Geometry check sheet. Reference: drawing and pictorial views, mm from the part's lowest x, y, z. A direction names the side the tool comes from. Round coordinates to 2 decimals unless told otherwise and drop trailing zeros. Loops run counter-clockwise (first coordinate to the right, second up) from the corner with the lowest first, then second, coordinate; pieces in that order, holes last. Notation, with made-up numbers: (-9, 39.5) -> (10, 39.5) arc R17 ccw to (10, 71.5) -> close; hole circle Ø5 at (77.5, 32.5). An arc over 180 degrees is marked (long way). Write item = value, one per line.
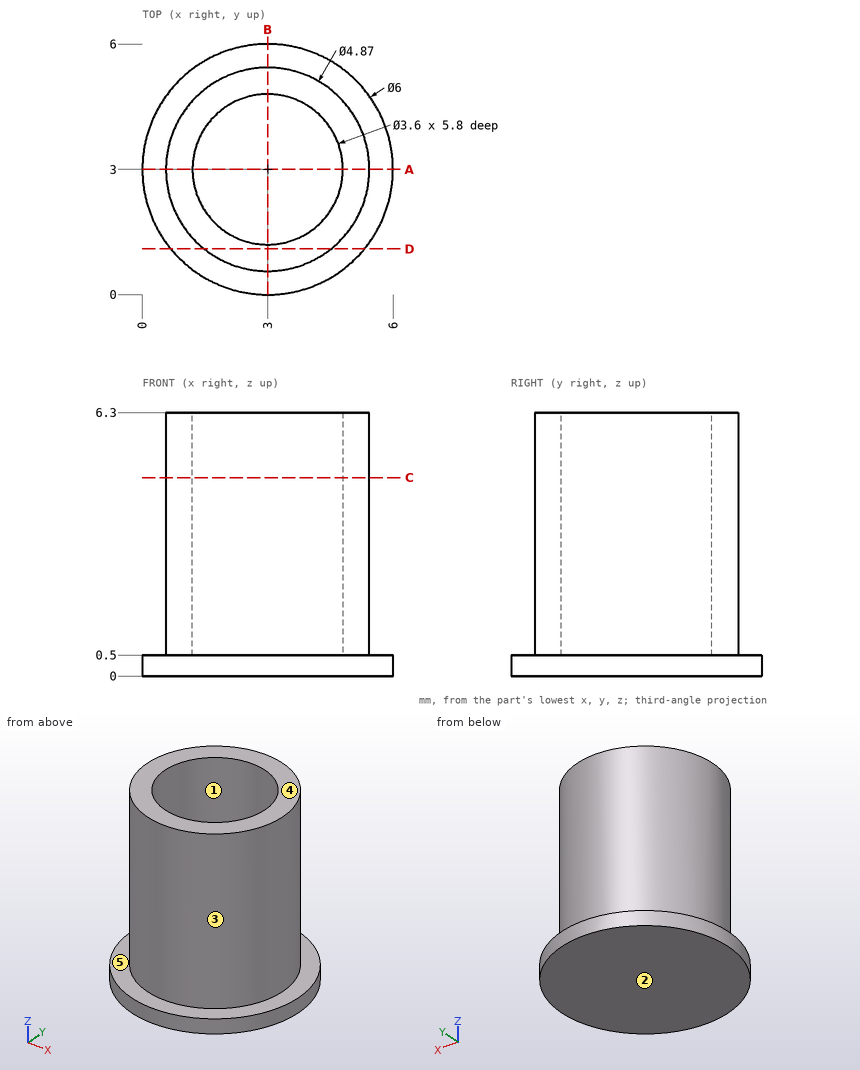
(1) Sectioned sample at D-D, the plane y = 1.1. Record the cut outline in (x, z).
Filled sheet:
outline = (0.68, 0) -> (5.32, 0) -> (5.32, 0.5) -> (4.52, 0.5) -> (4.52, 6.3) -> (1.48, 6.3) -> (1.48, 0.5) -> (0.68, 0.5) -> close
(2) Go/stop test with flat-tipped pins: pin 1 Ø1.5 at (x, y) = (3.5, 3) entering from +Z; pin 2 Ø3 at (y, z) = (5.5, 3.5) entering from -X; pin 3 Ø3 at (x, z) = (1, 5) entering from -Y. Record where each tip stops, or that it passes through.
Filled sheet:
pin_1 = 0.5
pin_2 = 0.78
pin_3 = 0.62
(3) Sectioned sample at C-C, the plane z = 4.75. Record the cut outline in (x, y) (3 decimals).
Filled sheet:
outline = circle Ø4.87 at (3, 3); hole circle Ø3.6 at (3, 3)
(4) Sectioned sample at A-A, the plane y = 3. Record the cut outline in (x, z) (3 decimals).
Filled sheet:
outline = (0, 0) -> (6, 0) -> (6, 0.5) -> (5.435, 0.5) -> (5.435, 6.3) -> (4.8, 6.3) -> (4.8, 0.5) -> (1.2, 0.5) -> (1.2, 6.3) -> (0.565, 6.3) -> (0.565, 0.5) -> (0, 0.5) -> close
(5) Draft check along X on the marked faces 1, 2 and 3. Enter one of: released by +X, released by -X, zero draft, split by the parting line, or undercut.
Filled sheet:
face_1 = undercut
face_2 = zero draft
face_3 = split by the parting line
(6) Material ranges on probe 1 along Y at (x, z) = (3, 1.7) (3 decimals); probe 2 along Z at (x, y) = (4.8, 1.05); probe 3 along X at (y, z) = (1.75, 1.75), recorded low to high. Write a range as from..to.
Filled sheet:
probe_1 = 0.565..1.2, 4.8..5.435
probe_2 = 0..0.5
probe_3 = 0.91..1.7, 4.3..5.09
(7) Set-up check for the marked faces 4 and 5: record each of +Z, -Z, +X, -X, +Y, -Y from which the full face is reachable in a straight line by a thin tool's end or side.
Filled sheet:
face_4 = +Z, +X, -X, +Y, -Y
face_5 = +Z
